Drawing for the job (mm, zero at the part's lowest x, y, z). A direction names the side the tool comes from. Coordinates: 2 decimals unless noted, no trailing zeros. Write each loop counter-clockwise with the first axis right and the second up, starting at its lowest first coordinate (ties: lowest second). Pieces come first, ordered by that corner, then holes. Notation, with made-up numbers: (52, -7.75) -> (65, -7.75) arc R26 ccw to (65, 9.25) -> close; hole circle Ø1 at (49, 53). An arc over 180 degrees is marked (long way). Write item = value, one per line. Start each with the question number.
Q1. Probe line 1 (X direction, y = 49, z = 15); line 2 (Y direction, x = 12, z = 20.25); line 3 (Z direction, x = 53.5, y = 63). List the from-to ranges inside material, lowest first.
Q2. Band-saw the part on B-B, the plane x = 10. List the corners of the cut face in (y, z).
Q3. Band-saw the part on A-A, the plane z = 19. List the corners of the cut face in (x, y).
Q4. Pin check, flat tips, straight feed: P1, Ø1.5, axis at x = 39, z = 20.5, coming from the -Y side; P2, Ø17.5, axis at x = 26, y = 24, coming from the +Z side; P3, Ø2, axis at x = 12.5, y = 1.5, coming from the -Z side; P4, Ø3, axis at x = 16, z = 2, coming from the -Y side. Stop position of each tip, or through.
Q5. Band-saw the part on C-C, the plane y = 46. List the corners of the cut face in (x, z).
Q6. Band-saw the part on D-D, the plane z = 6. List the corners of the cut face in (x, y) (1 decimal).
Q7. Pull direction X, two halves, no side cores. Call the marked faces 3, 4 and 5: released by +X, released by -X, zero draft, split by the parting line, or undercut.
Q8. Tool access for the marked faces 1 and 2: list every direction of +Z, -Z, +X, -X, +Y, -Y with a clear straight run to the whole face (end or side of a thin tool).
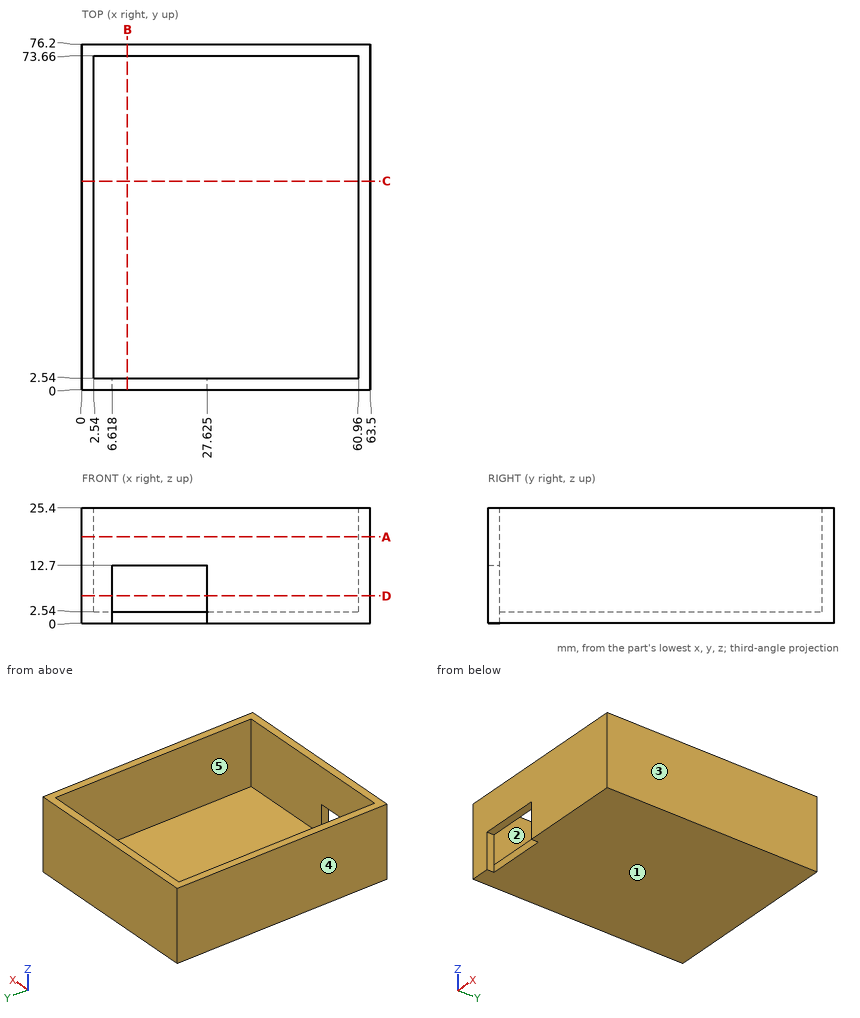
Ans:
q1.line_1 = 0 to 2.54, 60.96 to 63.5
q1.line_2 = 0 to 2.54, 73.66 to 76.2
q1.line_3 = 0 to 2.54
q2.outline = (0, 12.7) -> (2.54, 12.7) -> (2.54, 25.4) -> (0, 25.4) -> close; (2.54, 0) -> (76.2, 0) -> (76.2, 25.4) -> (73.66, 25.4) -> (73.66, 2.54) -> (2.54, 2.54) -> close
q3.outline = (0, 0) -> (63.5, 0) -> (63.5, 76.2) -> (0, 76.2) -> close; hole (2.54, 2.54) -> (60.96, 2.54) -> (60.96, 73.66) -> (2.54, 73.66) -> close
q4.P1 = 0
q4.P2 = 2.54
q4.P3 = 12.7
q4.P4 = 2.54
q5.outline = (0, 0) -> (63.5, 0) -> (63.5, 25.4) -> (60.96, 25.4) -> (60.96, 2.54) -> (2.54, 2.54) -> (2.54, 25.4) -> (0, 25.4) -> close
q6.outline = (0, 0) -> (6.6, 0) -> (6.6, 2.5) -> (2.5, 2.5) -> (2.5, 73.7) -> (61, 73.7) -> (61, 2.5) -> (27.6, 2.5) -> (27.6, 0) -> (63.5, 0) -> (63.5, 76.2) -> (0, 76.2) -> close
q7.face_3 = released by +X
q7.face_4 = released by -X
q7.face_5 = undercut
q8.face_1 = -Z, +X, -X, +Y, -Y
q8.face_2 = +Z
